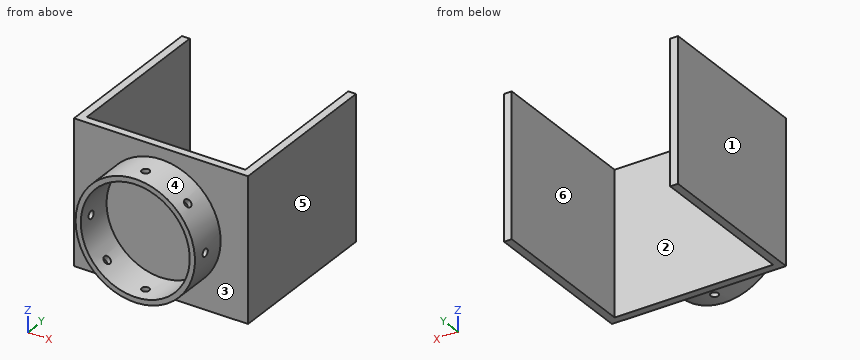
Autodesk Inventor part; units mm, degrees
ref_plane "YZ Plane" through (0, 0, 0) normal (1, 0, 0) x (0, 1, 0)
ref_plane "XZ Plane" through (0, 0, 0) normal (0, 1, 0) x (-1, 0, 0)
ref_plane "XY Plane" through (0, 0, 0) normal (0, 0, 1) x (1, 0, 0)
sketch "Sketch1" plane through (0, 0, 0) normal (0, 1, 0) x (-1, 0, 0)
  circle A0 centre (0, 0) radius 21
  circle A1 centre (0, 0) radius 23
  dimension "d0" = 42
  dimension "d1" = 2
extrude "Extrusion1" add sketch "Sketch1" along normal blind 15
sketch "Sketch2" plane through (0, 15, 0) normal (0, 1, 0) x (1, 0, 0)
  line L0 (26, -27.5) -> (-26, -27.5)
  line L1 (-26, 27.5) -> (26, 27.5)
  line L2 (26, -27.5) -> (-26, 27.5) construction
  line L3 (-26, -27.5) -> (26, 27.5) construction
  line L4 (-26, 27.5) -> (-29, 27.5)
  line L5 (-29, -27.5) -> (-26, -27.5)
  line L6 (26, 27.5) -> (29, 27.5)
  line L7 (29, -27.5) -> (26, -27.5)
  circle A0 centre (0, 0) radius 11.075
  line L8 (-30.543, 0) -> (-30.543, -27.5)
  line L9 (-30.543, -27.5) -> (-29, -27.5)
  line L10 (-30.543, 0) -> (-30.543, 27.5)
  line L11 (-30.543, 27.5) -> (-29.0865, 27.5)
  line L12 (30.543, 0) -> (30.543, 27.5)
  line L13 (30.543, 27.5) -> (29, 27.5)
  line L14 (30.543, 0) -> (30.543, -27.5)
  line L15 (30.543, -27.5) -> (29, -27.5)
  line L16 (30.543, -27.5) -> (33.543, -27.5)
  line L17 (33.543, -27.5) -> (33.543, 27.5)
  line L18 (33.543, 27.5) -> (30.543, 27.5)
  line L19 (-30.543, 27.5) -> (-33.543, 27.5)
  line L20 (-33.543, 27.5) -> (-33.543, -27.5)
  line L21 (-33.543, -27.5) -> (-30.543, -27.5)
  line L22 (-29.0865, 27.5) -> (-29, 27.5)
  line L23 (30.543, 27.5) -> (33.543, 27.5)
  line L24 (33.543, 27.5) -> (33.543, -27.5)
  line L25 (33.543, -27.5) -> (30.543, -27.5)
  line L26 (30.543, -27.5) -> (30.543, 27.5)
  line L27 (-33.543, 27.5) -> (-30.543, 27.5)
  line L28 (-30.543, 27.5) -> (-30.543, -27.5)
  line L29 (-30.543, -27.5) -> (-33.543, -27.5)
  line L30 (-33.543, -27.5) -> (-33.543, 27.5)
  dimension "d4" = 52
  dimension "d6" = 3
  dimension "d7" = 3
  dimension "d21" = 22.15
  dimension "d23" = 30.543
  dimension "d24" = 3
extrude "Extrusion2" add sketch "Sketch2" along normal blind 3 contours L0 L5 L9 L8 L10 L11 L22 L4 L1 L6 L13 L12 L14 L15 L7 | A0
sketch "Sketch3" plane through (0, 0, 0) normal (1, 0, 0) x (0, 1, 0)
  circle A0 centre (6, 0) radius 1.5
  line L0 (0, 21) -> (0, -21)
  point P0 (0, 0)
  dimension "d14" = 3
  dimension "d15" = 6
extrude "Extrusion4" cut sketch "Sketch3" along normal up to surface
pattern_circular "Circular Pattern1" count 8 over 360 about axis through (0, 0, 0) along (0, 1, 0) of "Extrusion4"
extrude "Extrusion5" add sketch "Sketch2" along normal blind 63 contours L14 L12 L18 L17 L16 | L21 L20 L19 L10 L8
properties part number "baseatas" material "Aluminum 6061"
The model under review builds one solid part; all positions refer to its coordinate system, in mm. Face numbers are marked on the shaded views. A direction names the side the tool comes from. Round coordinates to 2 decimals unless told otherwise and drop trailing zeros. Loops run counter-clockwise (first coordinate to the right, second up) from the corner with the lowest first, then second, coordinate; pieces in that order, holes last. Notation, with made-up numbers: M 28.5,43 L 66.5,43 A17 ccw 66.5,69 Z; hole C -9.5,-33.5 d10. An arc over 180 degrees is marked long. Write item = value, one per line.
Item 1: The part is to be moulded in two halves that separate along X. For the marked faces 1, 2 and 3, say which applies: released by +X, released by -X, zero draft, split by the parting line, or undercut.
Return value:
face_1 = released by -X
face_2 = undercut
face_3 = zero draft
Item 2: For line 1 (X direction, y = 54, z = -9.5); line 2 (Y direction, x = 0, z = -21.65); line 3 (Z direction, x = -1, y = 9.5), list the stretches that pass through material, from the lowest coordinate up. Write a range as [from, to].
Return value:
line_1 = [-33.54, -30.54], [30.54, 33.54]
line_2 = [0, 4.5], [7.5, 18]
line_3 = [-22.98, -20.98], [20.98, 22.98]
Item 3: Take a section at C-C on x = 0. Write out the cut boundary in (y, z), then the cut area to 3 significant figures.
Return value:
outline = M 0,-23 L 4.5,-23 L 4.5,-21 L 0,-21 Z; M 0,21 L 4.5,21 L 4.5,23 L 0,23 Z; M 7.5,-23 L 15,-23 L 15,-27.5 L 18,-27.5 L 18,27.5 L 15,27.5 L 15,23 L 7.5,23 L 7.5,21 L 15,21 L 15,-21 L 7.5,-21 Z
area = 213 mm2
Item 4: Take a section at B-B on y = 44. Write out the cut boundary in (x, z).
Return value:
outline = M -33.54,-27.5 L -30.54,-27.5 L -30.54,27.5 L -33.54,27.5 Z; M 30.54,-27.5 L 33.54,-27.5 L 33.54,27.5 L 30.54,27.5 Z
Item 5: Take a section at A-A on z = 0. Write out the cut boundary in (x, y).
Return value:
outline = M -33.54,15 L -23,15 L -23,7.5 L -21,7.5 L -21,15 L 21,15 L 21,7.5 L 23,7.5 L 23,15 L 33.54,15 L 33.54,78 L 30.54,78 L 30.54,18 L -30.54,18 L -30.54,78 L -33.54,78 Z; M -23,0 L -21,0 L -21,4.5 L -23,4.5 Z; M 21,0 L 23,0 L 23,4.5 L 21,4.5 Z
Item 6: Insertion check: P1, Ø4, axis at y = 6, z = 0, coming from the -X side; P2, Ø1.8, axis at x = 0, y = 6, coming from the -Z side; P3, Ø16.5, axis at x = 5.5, z = 0, coming from the -Y side; P4, Ø1.5, axis at x = 20.5, z = 19.5, coming from the +Y side. Each pin has a flat end and moves straight along its axis. Give the tip position at first contact, or say it passes through.
Return value:
P1 = -23
P2 = through
P3 = 15
P4 = 18
Item 7: Take a section at D-D on y = 6. State how many separate pieces and enclosed holes the cut face has, then the cut area to 3 significant figures.
Return value:
separate_pieces = 8
enclosed_holes = 0
area = 228 mm2
Item 8: Machinability: for the marked faces 4, 5 and 6, which of the approach directions +Z, -Z, +X, -X, +Y, -Y give a long, thin tool a straight path to every point of the face, cutting with its end or side? Answer none if there is none.
Return value:
face_4 = -Y
face_5 = +Z, -Z, +X, +Y, -Y
face_6 = +Z, -Z, +Y
